from build123d import *

# Parameters (mm, degrees)
BOSS_EXTRUDE2_DEPTH      = 82.5
BOSS_EXTRUDE2_DEPTH_BACK = 82.5
SKETCH4_R                = 3.175
BOSS_EXTRUDE3_DEPTH      = 12.7


with BuildPart() as part:
    # Sketch3 → Boss-Extrude2 (new body, two sides)
    with BuildSketch(Plane.XY) as boss_extrude2_sk:
        Polygon((-5.55625, -3.207902433), (0, -6.415804866), (5.55625, -3.207902433), (5.55625, 3.207902433), (0, 6.415804866), (-5.55625, 3.207902433), align=None)
    extrude(amount=BOSS_EXTRUDE2_DEPTH)
    extrude(boss_extrude2_sk.sketch, amount=-BOSS_EXTRUDE2_DEPTH_BACK)

    # Sketch4 → Boss-Extrude3 (add)
    with BuildSketch(Plane.XY.offset(-82.5)):
        Circle(SKETCH4_R)
    extrude(amount=-BOSS_EXTRUDE3_DEPTH)


solid = part.part
Build history of the part. All positions in model axes, mm. A direction names the side the tool comes from. Round coordinates to 2 decimals unless told otherwise and drop trailing zeros. Loops run counter-clockwise (first coordinate to the right, second up) from the corner with the lowest first, then second, coordinate; pieces in that order, holes last. Notation, with made-up numbers: (1, 6.5) -> (13, 6.5) arc R14 ccw to (13, 11.5) -> close; hole circle Ø8 at (-2, -17). An arc over 180 degrees is marked (long way). One line per item, written item: value. Start each with the question number.
Q1. Drop flat-ended pins along their axis: pin 1 Ø1 at (x, z) = (-3, -52) entering from +Y; pin 2 Ø2 at (x, z) = (-3, -34) entering from +Y; pin 3 Ø3 at (x, y) = (0.5, -5) entering from -Z. Give the stop position or say it passes through.
Q2. Probe line 1 along Y through (x, z) = (-1.5, 56.5); line 2 along Z through (x, y) = (4.75, 2.25); line 3 along Y through (x, z) = (-1.25, -85). List the from-to ranges inside material, lowest first.
Q3. Cut at B-B on y = 0. List the corners of the cut face in (x, z) (3 decimals).
Q4. 3-axis set-ups, long thin cutter, end or side, ignore diameter. For faces 1 (the face through (-0.69, -3.1, -88.76)), 2 (the face through (2.8, 4.8, 1.2)): which of +Z, -Z, +X, -X, +Y, -Y reach the whole face in a straight line?
Q5. Cut at A-A on z = 17. List the corners of the cut face in (x, y).
Computed:
1. pin 1: y = 4.97
1. pin 2: y = 5.26
1. pin 3: z = -82.5
2. line 1: -5.55 to 5.55
2. line 2: -82.5 to 82.5
2. line 3: -2.92 to 2.92
3. outline: (-5.556, -82.5) -> (-3.175, -82.5) -> (-3.175, -95.2) -> (3.175, -95.2) -> (3.175, -82.5) -> (5.556, -82.5) -> (5.556, 82.5) -> (-5.556, 82.5) -> close
4. face 1: -Z
4. face 2: +Z, -Z, +X, +Y
5. outline: (-5.56, -3.21) -> (0, -6.42) -> (5.56, -3.21) -> (5.56, 3.21) -> (0, 6.42) -> (-5.56, 3.21) -> close
